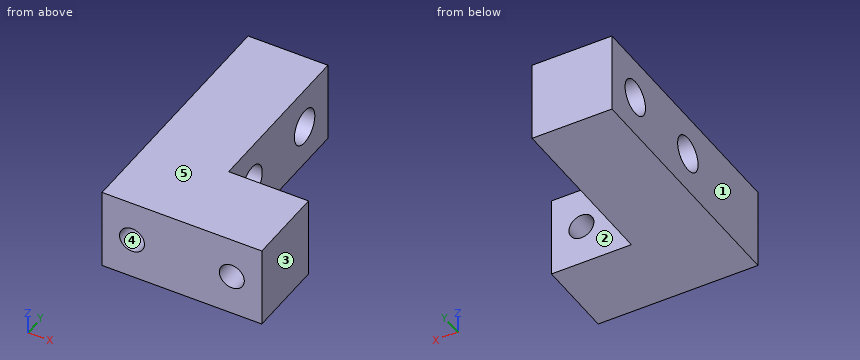
```python
from build123d import *

# Parameters (mm, degrees)
ESQUISSE1_W             = 16
ESQUISSE1_H             = 25
BOSS_EXTRU_1_DEPTH      = 8.1
ESQUISSE2_R             = 1.25
ENL_V_MAT_EXTRU_1_DEPTH = 8
ESQUISSE3_R             = 1.75
ENL_V_MAT_EXTRU_2_DEPTH = 8
ESQUISSE4_W             = 8
ESQUISSE4_H             = 17
ENL_V_MAT_EXTRU_3_DEPTH = 31.767027806


with BuildPart() as part:
    # Esquisse1 → Boss.-Extru.1 (new body)
    with BuildSketch(Plane.XY):
        with Locations((8, 12.5)):
            Rectangle(ESQUISSE1_W, ESQUISSE1_H)
    extrude(amount=BOSS_EXTRU_1_DEPTH)

    # Esquisse2 → Enlèv. mat.-Extru.1 (cut)
    with BuildSketch(Plane.XZ):
        with Locations(Location((3, 4.05, 0), (0, 0, 270))):
            Circle(ESQUISSE2_R)
        with Locations(Location((13, 4.05, 0), (0, 0, 90))):
            Circle(ESQUISSE2_R)
    extrude(amount=-ENL_V_MAT_EXTRU_1_DEPTH, mode=Mode.SUBTRACT)

    # Esquisse3 → Enlèv. mat.-Extru.2 (cut)
    with BuildSketch(Plane.ZY):
        with Locations((4.05, 21)):
            Circle(ESQUISSE3_R)
        with Locations((4.05, 12)):
            Circle(ESQUISSE3_R)
    extrude(amount=-ENL_V_MAT_EXTRU_2_DEPTH, mode=Mode.SUBTRACT)

    # Esquisse4 → Enlèv. mat.-Extru.3 (cut, through all)
    with BuildSketch(Plane.XY.offset(8.1)):
        with Locations((12, 16.5)):
            Rectangle(ESQUISSE4_W, ESQUISSE4_H)
    extrude(amount=-ENL_V_MAT_EXTRU_3_DEPTH, mode=Mode.SUBTRACT)


solid = part.part
```
Can you work these out from the model? Positions are in its coordinate system, mm. Face numbers are marked on the shaded views. A direction names the side the tool comes from. Coordinates: 2 decimals unless noted, no trailing zeros. Loops run counter-clockwise (first coordinate to the right, second up) from the corner with the lowest first, then second, coordinate; pieces in that order, holes last. Notation, with made-up numbers: (24, 27) - (81, 27) arc R28 ccw to (81, 50) - close; hole circle Ø4 at (7, 42.5). An arc over 180 degrees is marked (long way). Use a Markdown table: item, result.
Item 1: I want a section at A-A on y = 21. Please give me the cut outline in (x, z), and give its area (3 significant figures).
Numbers:
| item | result |
|---|---|
| outline | (0, 0) - (8, 0) - (8, 2.3) - (0, 2.3) - close; (0, 5.8) - (8, 5.8) - (8, 8.1) - (0, 8.1) - close |
| area | 36.8 mm2 |
Item 2: Will these pins go through, and if not, where does the flat tip stop? pin 1 (4 mm diameter, centred on x = 13, z = 4.05, fed in from -Y); pin 2 (1 mm diameter, centred on y = 19.5, z = 7, fed in from +X); pin 3 (2.5 mm diameter, centred on x = 10.5, z = 4.5, fed in from +Y).
Numbers:
| item | result |
|---|---|
| pin 1 | stops at y = 0 |
| pin 2 | stops at x = 8 |
| pin 3 | stops at y = 8 |
Item 3: We'd pull the mould along X, two halves only. Please class the marked faces 3, 4 and 5: released by +X, released by -X, zero draft, split by the parting line, or undercut.
Numbers:
| item | result |
|---|---|
| face 3 | released by +X |
| face 4 | undercut |
| face 5 | zero draft |
Item 4: If I drill on probe 1 along Y at (x, z) = (5.75, 4.05); probe 2 along X at (y, z) = (2.5, 4.05); probe 3 along Y at (x, z) = (3.25, 4.05), over which ranges is the centre line in solid material (lowest first)? Write a range as from..to.
Numbers:
| item | result |
|---|---|
| probe 1 | y = 0..10.25, 13.75..19.25, 22.75..25 |
| probe 2 | x = 0..1.75, 4.25..11.75, 14.25..16 |
| probe 3 | y = 8..10.25, 13.75..19.25, 22.75..25 |
Item 5: For the marked faces 1 and 2, which set-ups out of +Z, -Z, +X, -X, +Y, -Y let a thin tool reach every point of the face, with its end or its side?
Numbers:
| item | result |
|---|---|
| face 1 | +Z, -Z, -X, +Y, -Y |
| face 2 | +Z, -Z, +X, +Y |
Item 6: I want a section at C-C on z = 4.05. Please give me the cut outline in (x, y), and give its area (3 significant figures).
Numbers:
| item | result |
|---|---|
| outline | (0, 0) - (1.75, 0) - (1.75, 8) - (4.25, 8) - (4.25, 0) - (11.75, 0) - (11.75, 8) - (8, 8) - (8, 10.25) - (0, 10.25) - close; (0, 13.75) - (8, 13.75) - (8, 19.25) - (0, 19.25) - close; (0, 22.75) - (8, 22.75) - (8, 25) - (0, 25) - close; (14.25, 0) - (16, 0) - (16, 8) - (14.25, 8) - close |
| area | 168 mm2 |
Item 7: I want a section at D-D on x = 13. Please give me the cut outline in (y, z).
Numbers:
| item | result |
|---|---|
| outline | (0, 0) - (8, 0) - (8, 2.8) - (0, 2.8) - close; (0, 5.3) - (8, 5.3) - (8, 8.1) - (0, 8.1) - close |
Item 8: I want a section at B-B on x = 3. Please give me the cut outline in (y, z), and give its area (3 significant figures).
Numbers:
| item | result |
|---|---|
| outline | (0, 0) - (25, 0) - (25, 8.1) - (0, 8.1) - (0, 5.3) - (8, 5.3) - (8, 2.8) - (0, 2.8) - close; hole circle Ø3.5 at (12, 4.05); hole circle Ø3.5 at (21, 4.05) |
| area | 163 mm2 |
